Could you check a few things on this model? Use its own coordinates, in mm. Give positions to 0.01 mm unless a question says otherwise; leave off trailing zeros. Loops run counter-clockwise (first coordinate to the right, second up) from the corner with the lowest first, then second, coordinate; pieces in that order, holes last. Notation, with made-up numbers: M 34,-21.5 L 48,-21.5 A5 cw 48,-17.5 Z; hole C 22.5,45 d4. An arc over 180 degrees is marked long. Answer in a Markdown table with one row per item. Add a question column.
1. I'm going to push flat-ended pins straight in: pin 1 Ø0.6 at (y, z) = (-1, -18) entering from +X; pin 2 Ø0.6 at (y, z) = (-0.5, -17) entering from -X. Where does each tip first touch, or does it pass through?
2. If we section it at C-C on y = -0.9: List the corners of the cut face in (x, z) for me (3 decimals).
3. I need wall thicknesses on line 1 along Z through (x, y) = (0, -0.95); line 2 along Z through (x, y) = (-4.5, -0.9); line 3 along X through (y, z) = (-0.2, -3). Which ranges of each line are inside material? Lowest first, please. Write a range as from..to.
4. If we section it at A-A on z = 0: List the corners of the cut face in (x, y) for me.
5. If we section it at B-B on x = -8: List the corners of the cut face in (y, z) for me, then the cut area to 3 significant figures.
```python
from build123d import *

# Parameters (mm, degrees)
F0_R     = 0.95
F1_DEPTH = 1.3


# Not quite as in the source:
# - ends of sketch curves that miss each other by under 0.0002 mm in the source are joined


with BuildPart() as f1:
    # F0 (on Front) → F1 (new body)
    with BuildSketch(Plane.XZ):
        with BuildLine():
            ThreePointArc((-2.631999982, -16.2380748888), (2.5478e-06, 16.45), (2.631994952, -16.2380757041))
            Line((2.631994952, -16.2380757041), (2.632, -20.148075))
            Line((2.632, -20.148075), (7.1064, -20.148075))
            Line((7.1064, -20.148075), (10.639843, -15.19527))
            ThreePointArc((10.639843, -15.19527), (18.7183878017, 6.5879564678), (-5.9926e-06, 20.349999387))
            ThreePointArc((-5.9926e-06, 20.349999387), (-18.7183877489, 6.5879566442), (-10.6398432665, -15.1952704161))
            Line((-10.6398432665, -15.1952704161), (-7.1064, -20.148075))
            Line((-7.1064, -20.148075), (-2.632, -20.148075))
            Line((-2.632, -20.148075), (-2.631999982, -16.2380748888))
        make_face()
        with Locations((-5.0192, -18.155)):
            Circle(F0_R, mode=Mode.SUBTRACT)
        with Locations((5.0192, -18.155)):
            Circle(F0_R, mode=Mode.SUBTRACT)
    extrude(amount=F1_DEPTH)


solid = f1.part
```
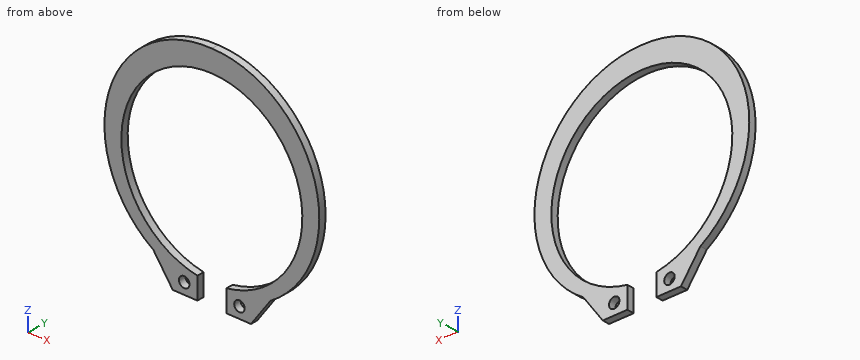
Results:
| question | item | result |
|---|---|---|
| 1 | pin 1 | x = 8.85 |
| 1 | pin 2 | x = -9.57 |
| 2 | outline | M -10.64,-15.195 L -7.106,-20.148 L -2.632,-20.148 L -2.632,-16.238 A16.45 cw long 2.632,-16.238 L 2.632,-20.148 L 7.106,-20.148 L 10.64,-15.195 A19.297 ccw 0,20.35 A19.297 ccw Z; hole C -5.019,-18.155 d1.9; hole C 5.019,-18.155 d1.9 |
| 3 | line 1 | 16.45..20.35 |
| 3 | line 2 | -20.15..-18.95, -17.36..-15.82, 15.82..19.87 |
| 3 | line 3 | -19.1..-16.17, 16.17..19.1 |
| 4 | outline | M -19.5,-1.3 L -16.45,-1.3 L -16.45,0 L -19.5,0 Z; M 16.45,-1.3 L 19.5,-1.3 L 19.5,0 L 16.45,0 Z |
| 5 | outline | M -1.3,-18.9 L 0,-18.9 L 0,-14.37 L -1.3,-14.37 Z; M -1.3,14.37 L 0,14.37 L 0,18.72 L -1.3,18.72 Z |
| 5 | area | 11.5 mm2 |
